Model file for the job. Use its own axes, mm. Give positions to 0.01 mm unless a question says otherwise; leave off trailing zeros. Order: outer loops, then holes, each group sorted by start corner. A loop starts at its lowest first (then second) coordinate and runs counter-clockwise, first axis right, second up. Notation, with made-up numbers: (45, 9) - (98, 9) arc R14 ccw to (98, 32) - close; hole circle Ø6 at (-28.5, 61.25). An arc over 180 degrees is marked (long way). Return JSON: item names as keys, results as strings. Group by question number.
from build123d import *

# Parameters (mm, degrees)
SKETCH2_R           = 11
SKETCH2_R_2         = 2.5
BOSS_EXTRUDE1_DEPTH = 4
CHAMFER1_SIZE       = 6.82619664
CHAMFER1_SIZE_2     = 2


with BuildPart() as part:
    # Sketch2 → Boss-Extrude1 (new body)
    with BuildSketch(Plane.XY):
        Polygon((80.138070711, -30), (69.467402807, 9.823474767), (-105, 9.823474767), (-105, -30), align=None)
        with Locations((35, -5)):
            Circle(SKETCH2_R, mode=Mode.SUBTRACT)
        with Locations((-65, -5)):
            Circle(SKETCH2_R, mode=Mode.SUBTRACT)
        with Locations((-92, -16)):
            Circle(SKETCH2_R_2, mode=Mode.SUBTRACT)
        with Locations((0, -16)):
            Circle(SKETCH2_R_2, mode=Mode.SUBTRACT)
        with Locations((-99, -0.176525233)):
            Circle(SKETCH2_R_2, mode=Mode.SUBTRACT)
        with Locations((-33, -1.453163789)):
            Circle(SKETCH2_R_2, mode=Mode.SUBTRACT)
        with Locations((55, -1.453163789)):
            Circle(SKETCH2_R_2, mode=Mode.SUBTRACT)
    extrude(amount=BOSS_EXTRUDE1_DEPTH)

    # Chamfer1
    # the kernel refuses this chamfer: 6.82619664, 2 mm, written as the material it takes off along each edge
    with BuildSketch(Plane(origin=(84.724761545, -47.117763232, 0), x_dir=(0.010461335179728238, 0.0028031063131594876, 0.9999413498107049), z_dir=(-0.25881904510252185, 0.965925826289068, 0))) as chamfer1_piece_1:
        Polygon((CHAMFER1_SIZE * 0.999941349797, -CHAMFER1_SIZE * 0.0108303711267), (-CHAMFER1_SIZE_2 * 0.0108303711269, -CHAMFER1_SIZE_2 * 0.999941349811), (0, 0), align=None)
    extrude(amount=76.67151992, mode=Mode.SUBTRACT)


solid = part.part
(1) Slice it at C-C (x = 0). Give the cut face in (y, z), and give its area (3 significant figures).
(2) Drop flat-ended pins along their axis: pin 1 Ø3 at (x, y) = (-33, -1.45) entering from +Z; pin 2 Ø2 at (y, z) = (-8.5, 1.5) entering from +X; pin 3 Ø1.5 at (y, z) = (-13.5, 0.5) entering from +X; pin 4 Ø2 at (y, z) = (3.5, 3) entering from +X. Give the stop position or say it passes through.
(3) Slice it at B-B (z = 3.25). Give the cut face in (x, y), and give its area (3 significant figures).
(4) Drill centre lines: L1, parallel to Y at x = -33, z = 3.2; L2, parallel to Y at x = -99, z = 3.1; L3, parallel to X at y = -19, z = 0.8. Where is each one in solid material? Low to high.
(5) Pull direction Y, two halves, no side cores. Call faces 1 (the face through (73.422, -10.367, 2.028)), 2 (the face through (24, -5, 2)), 3 (the face through (-105, -10, 2)): released by +Y, released by -Y, zero draft, split by the parting line, or undercut.
(6) Slice it at A-A (x = -65). Give the cut face in (y, z).
Result set:
{
 "1": {"outline": "(-30, 0) - (-18.5, 0) - (-18.5, 4) - (-30, 4) - close; (-13.5, 0) - (9.82, 0) - (9.82, 4) - (-13.5, 4) - close", "area": "139 mm²"},
 "2": {"pin 1": "passes through", "pin 2": "stops at x = 73.17", "pin 3": "stops at x = 74.1", "pin 4": "stops at x = 70.41"},
 "3": {"outline": "(-105, -30) - (79.05, -30) - (68.38, 9.82) - (-105, 9.82) - close; hole circle Ø5 at (-99, -0.18); hole circle Ø5 at (-92, -16); hole circle Ø22 at (-65, -5); hole circle Ø5 at (-33, -1.45); hole circle Ø5 at (0, -16); hole circle Ø22 at (35, -5); hole circle Ø5 at (55, -1.45)", "area": "6,260 mm²"},
 "4": {"L1": "y = -30 to -3.95, 1.05 to 9.82", "L2": "y = -30 to -2.68, 2.32 to 9.82", "L3": "x = -105 to 75.36"},
 "5": {"face 1": "released by +Y", "face 2": "undercut", "face 3": "zero draft"},
 "6": {"outline": "(-30, 0) - (-16, 0) - (-16, 4) - (-30, 4) - close; (6, 0) - (9.82, 0) - (9.82, 4) - (6, 4) - close"}
}
